Here's the drawing with two shaded views (mm, measured from the low corner). I have some questions. A direction names the side the tool comes from. Coordinates: 2 decimals unless noted, no trailing zeros. Order: outer loops, then holes, each group sorted by start corner. A loop starts at its lowest first (then second) coordinate and runs counter-clockwise, first axis right, second up. Notation, with made-up numbers: M 24.25,69 L 51.25,69 A10 cw 51.25,79 Z; hole C -13.75,-3.5 d3. An arc over 180 degrees is marked long. Put each result on its own line as item: value. Start each with the question number.
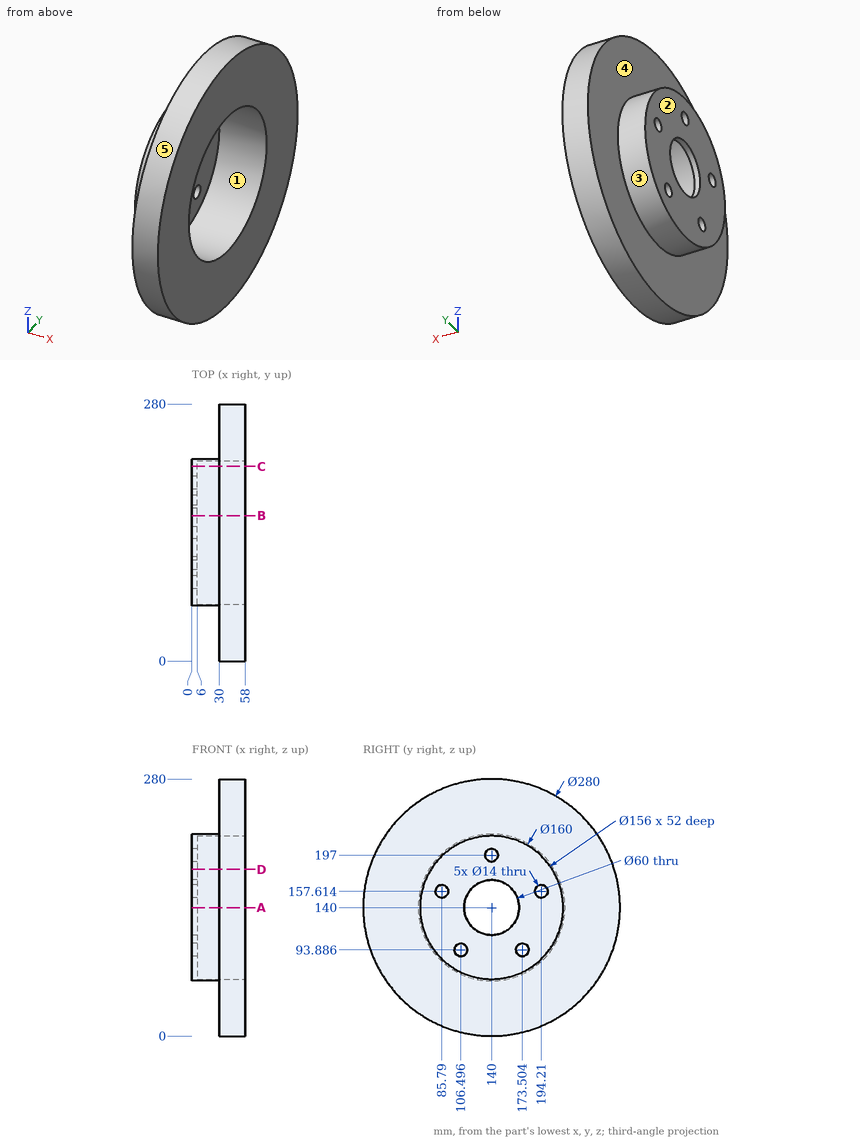
Item 1: If we section it at D-D on z = 181.5: Write out the boundary of the cut face in (x, y).
Item 2: If we section it at A-A on z = 140: Write out the boundary of the cut face in (x, y).
Item 3: For pin 1 Ø3 at (x, z) = (38, 161.5) entering from +Y; pin 2 Ø4 at (x, y) = (21.5, 90) entering from +Z; pin 3 Ø8 at (x, z) = (12.5, 137.5) entering from +Y; pin 4 Ø4 at (x, y) = (27, 224) entering from -Z, each with a flat end and sliding along its axis, tell me the tip position at first contact or that it passes through.
Item 4: If we mould it in two halves opening along Y, with no side actions, what happens to the marked faces 1, 2 and 3? For each: released by +Y, released by -Y, zero draft, split by the parting line, or undercut.
Item 5: If we section it at C-C on y = 212: Write out the boundary of the cut face in (x, z), then the cut area to 3 significant figures.
Item 6: If we section it at B-B on y = 158.5: Write out the boundary of the cut face in (x, z), then the cut area to 3 significant figures.
Item 7: I need wall thicknesses on probe 1 along Z at (x, y) = (3.7, 140); probe 2 along Y at (x, z) = (37, 140). Which ranges of each line are inside material? Lowest first, please.
Item 8: For the marked faces 4 and 5, which set-ups out of +Z, -Z, +X, -X, +Y, -Y let a thin tool reach every point of the face, with its end or its side?
Geometry check:
1. outline: M 0,71.61 L 30,71.61 L 30,6.29 L 58,6.29 L 58,73.96 L 6,73.96 L 6,206.04 L 58,206.04 L 58,273.71 L 30,273.71 L 30,208.39 L 0,208.39 Z
2. outline: M 0,60 L 30,60 L 30,0 L 58,0 L 58,62 L 6,62 L 6,110 L 0,110 Z; M 0,170 L 6,170 L 6,218 L 58,218 L 58,280 L 30,280 L 30,220 L 0,220 Z
3. pin 1: stops at y = 278.56
3. pin 2: stops at z = 204
3. pin 3: stops at y = 220
3. pin 4: passes through
4. face 1: undercut
4. face 2: zero draft
4. face 3: split by the parting line
5. outline: M 0,105.13 L 30,105.13 L 30,19.93 L 58,19.93 L 58,110 L 6,110 L 6,170 L 58,170 L 58,260.07 L 30,260.07 L 30,174.87 L 0,174.87 Z
5. area: 5,700 mm²
6. outline: M 0,62.17 L 30,62.17 L 30,1.23 L 58,1.23 L 58,64.23 L 6,64.23 L 6,116.38 L 0,116.38 Z; M 0,163.62 L 6,163.62 L 6,215.77 L 58,215.77 L 58,278.77 L 30,278.77 L 30,217.83 L 0,217.83 Z
6. area: 4,280 mm²
7. probe 1: z = 60 to 110, 170 to 190, 204 to 220
7. probe 2: y = 0 to 62, 218 to 280
8. face 4: -X
8. face 5: +X, -X
